Geometry: final body of the model. Coordinates: model frame, mm. Face numbers are marked on the shaded views. A direction names the side the tool comes from. Give positions to 0.01 mm unless a question says otherwise; leave off trailing zeros. Write each loop counter-clockwise with the first axis right and the second up, starting at its lowest first coordinate (ties: lowest second). Pieces come first, ordered by that corner, then holes. Notation, with made-up numbers: M -5.75,15 L 22.25,15 A19 cw 22.25,38 Z; hole C 11,85.5 d5. An arc over 180 degrees is marked long. Answer as a JSON object with one key per item and string values.
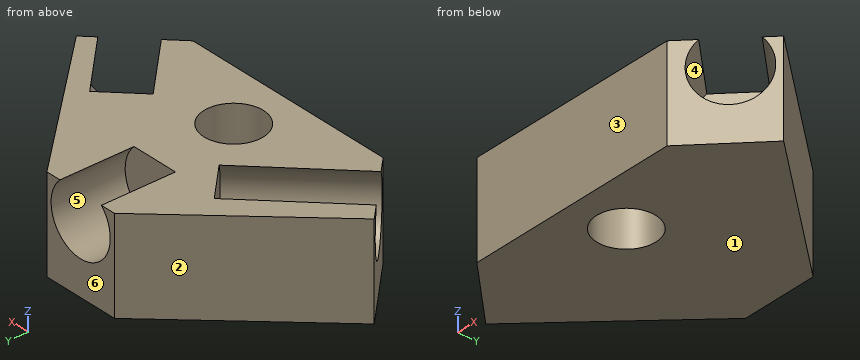
from build123d import *

# Parameters (mm, degrees)
F1_DEPTH = 19
F2_R     = 7
F3_DEPTH = 16
F4_R     = 7
F5_DEPTH = 25
F6_R     = 7
F7_DEPTH = 15
F8_R     = 6
F9_DEPTH = 19.001


with BuildPart() as f1:
    # F0 (on Top) → F1 (new body)
    with BuildSketch(Plane.XY):
        Polygon((-12.7437102583, 12.7121142558), (0, 0), (45, 0), (57.7437102583, 12.7121142558), (30.5, 42), (22.5, 42), (14.5, 42), align=None)
    extrude(amount=F1_DEPTH)

    # F2 (on face) → F3 (cut)
    with BuildSketch(Plane(origin=(22.4441456741, -22.4999306731, 0), x_dir=(0.7079839032, 0.7062285698, 0), z_dir=(0.7062285698, -0.7079839032, 0))):
        with Locations((41.6372567415, 14)):
            Circle(F2_R)
    extrude(amount=-F3_DEPTH, mode=Mode.SUBTRACT)

    # F4 (on face) → F5 (cut)
    with BuildSketch(Plane(origin=(0, 0, 0), x_dir=(0.7079839032, -0.7062285698, 0), z_dir=(-0.7062285698, -0.7079839032, 0))):
        with Locations((-9, 14)):
            Circle(F4_R)
    extrude(amount=-F5_DEPTH, mode=Mode.SUBTRACT)

    # F6 (on face) → F7 (cut)
    with BuildSketch(Plane(origin=(0, 42, 0), x_dir=(-1, 0, 0), z_dir=(0, 1, 0))):
        with Locations((-22.5, 14)):
            Circle(F6_R)
    extrude(amount=-F7_DEPTH, mode=Mode.SUBTRACT)

    # F8 (on face) → F9 (cut, through all)
    with BuildSketch(Plane.XY.offset(19)):
        with Locations((22.5, 11)):
            Circle(F8_R)
    extrude(amount=-F9_DEPTH, mode=Mode.SUBTRACT)


solid = f1.part
1) Set-up query: the marked faces 5 and 6. Return all of +Z, -Z, +X, -X, +Y, -Y with unobstructed straight access to the full face (end or side cutting, diameter ignored); none if empty.
Geometry check:
{"face 5": "+Y", "face 6": "+Z, -Z, +X, -X, +Y"}
2) Line query: line 1 (Y direction, x = 22.5, z = 8); line 2 (X direction, y = 19, z = 10.75); line 3 (X direction, y = 14, z = 9.75). Output: solid intervals per line, ascending. Write a range as from..to.
Geometry check:
{"line 1": "y = 0..5, 17..27", "line 2": "x = -6.89..-2.52, 15..41.39, 48.62..51.89", "line 3": "x = -11.55..-6.6, 9.11..17.3, 27.7..36.99, 52.7..56.55"}
3) Pull-direction query (Y, two-part tool) for the marked faces 1, 2, 3 and 4; classes: pulls with the +Y half, pulls with the -Y half, needs draft (parallel to the pull), parting line crosses it, or undercut.
Geometry check:
{"face 1": "needs draft", "face 2": "pulls with the +Y half", "face 3": "pulls with the -Y half", "face 4": "undercut"}
4) Cut plane D-D on y = 34. Return loops of the section in (x, z), and give its area (3 significant figures).
Geometry check:
{"outline": "M 7.06,0 L 37.94,0 L 37.94,19 L 27.4,19 A7 cw long 17.6,19 L 7.06,19 Z", "area": "446 mm2"}
5) Cut plane B-B on x = 22.5. Return loops of the section in (y, z), and give its area (3 significant figures).
Geometry check:
{"outline": "M 0,0 L 5,0 L 5,19 L 0,19 Z; M 17,0 L 42,0 L 42,7 L 27,7 L 27,19 L 17,19 Z", "area": "390 mm2"}
6) Cut plane A-A on z = 3.5. Return loops of the section in (x, y).
Geometry check:
{"outline": "M -12.74,12.71 L 0,0 L 45,0 L 57.74,12.71 L 30.5,42 L 14.5,42 Z; hole C 22.5,11 d12"}
7) Contact query for flat-ended pins moving along their axis: P1, Ø1.5, axis at x = 50, z = 14.5, coming from the -Y side; P2, Ø5, axis at y = 19.5, z = 8, coming from the +X side; P3, Ø8, axis at y = 20.5, z = 2.5, coming from the -X side. Output: stop coordinate, or through.
Geometry check:
{"P1": "stops at y = 17.96", "P2": "stops at x = 53.76", "P3": "stops at x = -9.22"}
8) Cut plane C-C on z = 12. Return loops of the section in (x, y).
Geometry check:
{"outline": "M -12.74,12.71 L -11.12,11.09 L 6.53,28.79 L 16.03,19.32 L -1.62,1.62 L 0,0 L 45,0 L 47.17,2.17 L 35.87,13.5 L 45.37,22.97 L 56.67,11.64 L 57.74,12.71 L 30.5,42 L 29.21,42 L 29.21,27 L 15.79,27 L 15.79,42 L 14.5,42 Z; hole C 22.5,11 d12"}
